```python
from build123d import *

# Parameters (mm, degrees)
SKIZZE1_R             = 8.5
GK_DEPTH              = 15.5
CUT_EXTRUDE_START     = -14
SKIZZE2_R             = 8.5
SKIZZE2_R_2           = 7.5
CUT_EXTRUDE_D15_DEPTH = 14
SKIZZE3_W             = 15
SKIZZE3_H             = 6
SW14_DEPTH            = 0.5
SKIZZE4_R             = 6
AU_ENGEWINDE_DEPTH    = 9
SKIZZE18_R            = 4.65
D9_3MM_DEPTH          = 28.290108098
SKIZZE19_R            = 6
KERNLOCH_D12_DEPTH    = 8
FASE_0_2MM_SIZE       = 0.2
FASE_0_5MM_SIZE       = 0.5


with BuildPart() as part:
    # Skizze1 → GK (new body)
    with BuildSketch(Plane(origin=(0, 0, 0), x_dir=(1, 0, 0), z_dir=(0, 1, 0))):
        with Locations(Location((0, 0, 0), (0, 0, 270))):
            Circle(SKIZZE1_R)
    extrude(amount=GK_DEPTH)

    # Skizze2 → D15 (cut)
    with BuildSketch(Plane(origin=(0, 15.5, 0), x_dir=(1, 0, 0), z_dir=(0, 1, 0)).offset(CUT_EXTRUDE_START)):
        with Locations(Location((0, 0, 0), (0, 0, 270))):
            Circle(SKIZZE2_R)
        with Locations(Location((0, 0, 0), (0, 0, 270))):
            Circle(SKIZZE2_R_2, mode=Mode.SUBTRACT)
    extrude(amount=CUT_EXTRUDE_D15_DEPTH, mode=Mode.SUBTRACT)

    # Skizze3 → SW14 (cut)
    with BuildSketch(Plane(origin=(7.5, 0, 0), x_dir=(0, 0, -1), z_dir=(1, 0, 0))):
        with Locations((0, 4.5)):
            Rectangle(SKIZZE3_W, SKIZZE3_H)
    sw14 = extrude(amount=-SW14_DEPTH, mode=Mode.SUBTRACT)

    # Spiegeln1: SW14 across plane
    add(sw14.mirror(Plane(origin=(0, 0, 0), x_dir=(0, 0, 1), z_dir=(1, 0, 0))), mode=Mode.SUBTRACT)

    # Skizze4 → Außengewinde (add)
    with BuildSketch(Plane.XZ):
        with Locations(Location((0, 0, 0), (0, 0, 270))):
            Circle(SKIZZE4_R)
    extrude(amount=AU_ENGEWINDE_DEPTH)

    # Skizze18 → D9,3mm (cut, through all)
    with BuildSketch(Plane.XZ.offset(9)):
        with Locations(Location((0, 0, 0), (0, 0, 270))):
            Circle(SKIZZE18_R)
    extrude(amount=-D9_3MM_DEPTH, mode=Mode.SUBTRACT)

    # Skizze19 → Kernloch D12 (cut)
    with BuildSketch(Plane(origin=(0, 15.5, 0), x_dir=(1, 0, 0), z_dir=(0, 1, 0))):
        with Locations(Location((0, 0, 0), (0, 0, 90))):
            Circle(SKIZZE19_R)
    extrude(amount=-KERNLOCH_D12_DEPTH, mode=Mode.SUBTRACT)

    # Fase 0,2mm
    fase_0_2mm_edges = [part.edges().sort_by_distance(p)[0] for p in [
        (0, 0, -8.5),
        (0, 1.5, -8.5),
        (0, 15.5, -7.5),
    ]]
    chamfer(fase_0_2mm_edges, length=FASE_0_2MM_SIZE)

    # Fase 0,5mm
    fase_0_5mm_edges = [part.edges().sort_by_distance(p)[0] for p in [
        (0, -9, 6),
        (0, 15.5, 6),
    ]]
    chamfer(fase_0_5mm_edges, length=FASE_0_5MM_SIZE)


solid = part.part
```
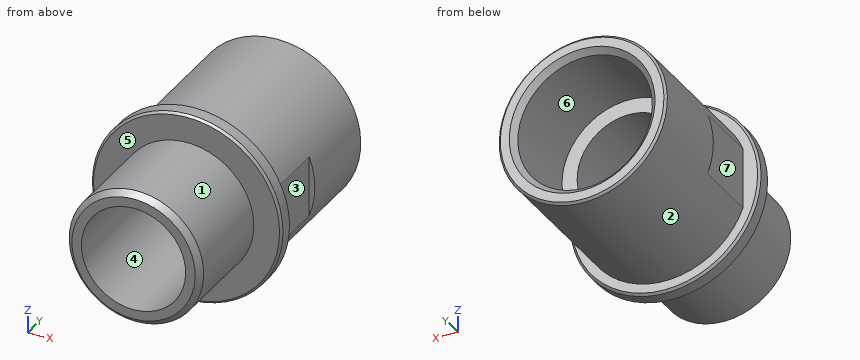
Build history of the part. All positions in model axes, mm. Face numbers are marked on the shaded views. A direction names the side the tool comes from. Give positions to 0.01 mm unless a question says otherwise; leave off trailing zeros. Loops run counter-clockwise (first coordinate to the right, second up) from the corner with the lowest first, then second, coordinate; pieces in that order, holes last. Notation, with made-up numbers: (-0.75, 60.25) - (39.25, 60.25) arc R25 ccw to (39.25, 96.25) - close; hole circle Ø5 at (74.5, 16). An arc over 180 degrees is marked (long way). Use a Markdown table: item, result.
(1) Band-saw the part on D-D (y = 8). Give the cut face in (x, z).
Taken from the geometry:
| item | result |
|---|---|
| outline | circle Ø15 at (0, 0); hole circle Ø12 at (0, 0) |
(2) Which spindle directions (+Z, -Z, +X, -X, +Y, -Y) get a long thin tool onto all of the face, cutting with end or side? Do the marked faces 1, 2, 3 and 4. Say none if no direction does.
Taken from the geometry:
| item | result |
|---|---|
| face 1 | -Y |
| face 2 | +Y |
| face 3 | +Z, -Z, +X |
| face 4 | +Y, -Y |
(3) Drop flat-ended pins along their axis: pin 1 Ø3.5 at (x, z) = (-2.5, -2) entering from +Y; pin 2 Ø0.6 at (x, z) = (-7.5, 0) entering from -Y; pin 3 Ø2.5 at (y, z) = (4.5, 0.5) entering from +X. Give the stop position or say it passes through.
Taken from the geometry:
| item | result |
|---|---|
| pin 1 | y = 7.5 |
| pin 2 | y = 0 |
| pin 3 | x = 7 |
(4) Pull direction Y, two halves, no side cores. Call the marked faces 5, 6 and 7: +Y half, -Y half, draft (parallel to the pull), parting line (faces both ways), or undercut.
Taken from the geometry:
| item | result |
|---|---|
| face 5 | -Y half |
| face 6 | draft |
| face 7 | undercut |
(5) Wall check: line 1 along X through (y, z) = (9.25, 0); line 2 along X through (y, z) = (1.25, 0); line 3 along Y through (x, z) = (-2.5, 4.25). Give the ranges that are in metal, low to high.
Taken from the geometry:
| item | result |
|---|---|
| line 1 | -7.5 to -6, 6 to 7.5 |
| line 2 | -8.5 to -4.65, 4.65 to 8.5 |
| line 3 | -9 to 7.5 |
(6) Band-saw the part on B-B (y = 2). Give the cut face in (x, z), and give its area (3 significant figures).
Taken from the geometry:
| item | result |
|---|---|
| outline | (-7, -2.69) arc R7.5 ccw to (7, -2.69) - (7, 2.69) arc R7.5 ccw to (-7, 2.69) - close; hole circle Ø9.3 at (0, 0) |
| area | 105 mm2 |
